Could you check a few things on this model? Use its own coordinates, in mm. Face numbers are marked on the shaded views. A direction names the side the tool comes from. Coordinates: 2 decimals unless noted, no trailing zeros. Loops run counter-clockwise (first coordinate to the right, second up) from the corner with the lowest first, then second, coordinate; pieces in that order, holes last. Notation, with made-up numbers: M -33.5,-40 L -12.5,-40 A11 ccw -12.5,-24 Z; hole C 53.5,-13.5 d11. An arc over 180 degrees is marked long. Write each question's results on one line, items separated by ' | '.
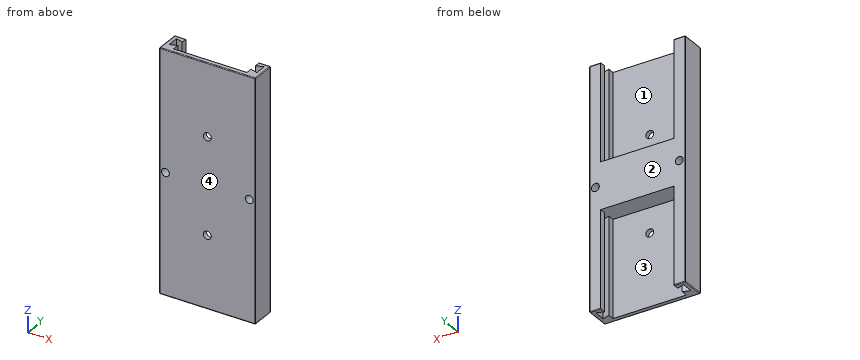
Autodesk Inventor part; units mm, degrees
ref_plane "YZ Plane" through (0, 0, 0) normal (1, 0, 0) x (0, 1, 0)
ref_plane "XZ Plane" through (0, 0, 0) normal (0, 1, 0) x (-1, 0, 0)
ref_plane "XY Plane" through (0, 0, 0) normal (0, 0, 1) x (1, 0, 0)
sketch "Sketch1" plane through (0, 0, 0) normal (0, 0, 1) x (1, 0, 0)
  line L0 (0, 0) -> (40, 0)
  line L1 (40, 0) -> (40, 10)
  line L2 (40, 10) -> (0, 10)
  line L3 (0, 10) -> (0, 0)
  dimension "d0" = 40
  dimension "d1" = 10
extrude "Extrusion1" add sketch "Sketch1" against normal blind 100
sketch "Sketch2" plane through (0, 0, 0) normal (0, 0, 1) x (1, 0, 0)
  line L0 (4.7, 1.898) -> (35.3, 1.898)
  line L1 (38.3, 8.5152) -> (38.3, 3.6828)
  line L2 (1.7, 8.5152) -> (1.7, 3.6828)
  line L3 (35.3, 7.5152) -> (38.3, 8.5152)
  line L4 (35.3, 7.5152) -> (35.3, 10)
  line L5 (35.3, 1.898) -> (35.3, 4.6828)
  line L6 (38.3, 3.6828) -> (35.3, 4.6828)
  line L7 (4.7, 7.5152) -> (1.7, 8.5152)
  line L8 (4.7, 10) -> (4.7, 7.5152)
  line L9 (4.7, 4.6828) -> (4.7, 1.898)
  line L10 (1.7, 3.6828) -> (4.7, 4.6828)
  line L11 (4.7, 10) -> (35.3, 10)
extrude "Extrusion2" cut sketch "Sketch2" against normal blind 40.3
sketch "Sketch3" plane through (0, 0, -100) normal (0, 0, -1) x (-1, 0, 0)
  line L0 (-35.3, 1.898) -> (-4.7, 1.898)
  line L1 (-1.7, 8.5152) -> (-1.7, 3.6828)
  line L2 (-38.3, 8.5152) -> (-38.3, 3.6828)
  line L3 (-4.7, 7.5152) -> (-1.7, 8.5152)
  line L4 (-4.7, 7.5152) -> (-4.7, 10)
  line L5 (-4.7, 1.898) -> (-4.7, 4.6828)
  line L6 (-1.7, 3.6828) -> (-4.7, 4.6828)
  line L7 (-35.3, 7.5152) -> (-38.3, 8.5152)
  line L8 (-35.3, 10) -> (-35.3, 7.5152)
  line L9 (-35.3, 4.6828) -> (-35.3, 1.898)
  line L10 (-38.3, 3.6828) -> (-35.3, 4.6828)
  line L11 (-35.3, 10) -> (-4.7, 10)
extrude "Extrusion3" cut sketch "Sketch3" against normal blind 40.3
sketch "Sketch5" plane through (4.7, 1.898, 0) normal (0, 1, 0) x (1, 0, 0)
  circle A0 centre (15.3, 30) radius 1.65
  line L0 (35.3, 0) -> (35.3, 100)
  circle A1 centre (15.3, 70) radius 1.65
  point P0 (-4.7, 0)
extrude "Extrusion5" cut sketch "Sketch5" against normal blind 5
fillet "Fillet1" radius 0.3 14 edges at (2.35, 10, -100) (37.65, 10, -100) (0, 5, -100) (0, 10, -50) (0, 0, -50) (20, 0, -100) (40, 5, -100) (0, 5, 0) (40, 10, -50) (40, 0, -50) (20, 0, 0) (40, 5, 0) (2.35, 10, 0) (37.65, 10, 0)
sketch "Sketch6" plane through (4.7, 10, -40.3) normal (0, 1, 0) x (1, 0, 0)
  line L0 (-4.4, -40) -> (-4.4, 59.4)
  line L1 (-4.7, 59.4) -> (-4.7, -40)
  line L2 (35.3, -40) -> (35.3, 59.4)
  circle A0 centre (32.8, 9.7) radius 1.65
  circle A1 centre (-2.2, 9.7) radius 1.65
  point P0 (-4.7, -40.3)
  dimension "d29" = 3.3
  dimension "d30" = 3.3
extrude "Extrusion6" cut sketch "Sketch6" against normal blind 10
properties part number "centralBody"
(1) Imagine slicing it at C-C, the plane z = -50. List the corners of the cut face in (x, y) for me.
Reported:
outline: M 0,0.3 A0.3 ccw 0.3,0 L 0.85,0 L 0.85,10 L 0.3,10 A0.3 ccw 0,9.7 Z; M 4.15,0 L 35.85,0 L 35.85,10 L 4.15,10 Z; M 39.15,0 L 39.7,0 A0.3 ccw 40,0.3 L 40,9.7 A0.3 ccw 39.7,10 L 39.15,10 Z
(2) Please list where these lines run through material, in increasing order: probe 1 along X at (y, z) = (8, -50); probe 2 along Z at (x, y) = (20, 1.45); probe 3 along X at (y, z) = (1.3, -70). Write a range as from..to.
Reported:
probe 1: x = 0..0.85, 4.15..35.85, 39.15..40 | probe 2: z = -100..-71.65, -68.35..-31.65, -28.35..0 | probe 3: x = 0..18.35, 21.65..40
(3) Which directions (+Z, -Z, +X, -X, +Y, -Y) give clear straight access to the entire face, cutting with the end or side of a thin tool? Please do the marked faces 3 and 4.
Reported:
face 3: -Z, +Y | face 4: +Z, -Z, +X, -X, -Y
(4) Will these pins go through, and if not, where does the flat tip stop? P1, Ø3, axis at x = 10.5, z = -28.5, coming from the +Y side; P2, Ø1.5, axis at x = 11, y = 4.5, coming from the -Z side; P3, Ø2.5, axis at y = 5.5, z = -17, coming from the -X side; P4, Ø2.5, axis at x = 26, y = 7, coming from the +Z side.
Reported:
P1: stops at y = 1.9 | P2: stops at z = -59.7 | P3: stops at x = 0 | P4: stops at z = -40.3
(5) Imagine slicing it at B-B, the plane x = 20. List the corners of the cut face in (y, z) for me, and give its area (3 significant figures).
Reported:
outline: M 0,-99.7 A0.3 ccw 0.3,-100 L 1.9,-100 L 1.9,-71.65 L 0,-71.65 Z; M 0,-68.35 L 1.9,-68.35 L 1.9,-59.7 L 10,-59.7 L 10,-40.3 L 1.9,-40.3 L 1.9,-31.65 L 0,-31.65 Z; M 0,-28.35 L 1.9,-28.35 L 1.9,0 L 0.3,0 A0.3 ccw 0,-0.3 Z | area: 334 mm2
(6) Imagine slicing it at A-A, the plane z = -70. List the corners of the cut face in (x, y) for me.
Reported:
outline: M 0,0.3 A0.3 ccw 0.3,0 L 18.35,0 L 18.35,1.9 L 4.7,1.9 L 4.7,4.68 L 1.7,3.68 L 1.7,8.52 L 4.7,7.52 L 4.7,10 L 0.3,10 A0.3 ccw 0,9.7 Z; M 21.65,0 L 39.7,0 A0.3 ccw 40,0.3 L 40,9.7 A0.3 ccw 39.7,10 L 35.3,10 L 35.3,7.52 L 38.3,8.52 L 38.3,3.68 L 35.3,4.68 L 35.3,1.9 L 21.65,1.9 Z
(7) If we mould it in two halves opening along X, with no side actions, what happens to the marked faces 1 and 2? For each: released by +X, released by -X, zero draft, split by the parting line, or undercut.
Reported:
face 1: undercut | face 2: zero draft
(8) Imagine slicing it at D-D, the plane y = 6. List the corners of the cut face in (x, z) for me, and give its area (3 significant figures).
Reported:
outline: M 0,-99.7 A0.3 ccw 0.3,-100 L 1.7,-100 L 1.7,-59.7 L 38.3,-59.7 L 38.3,-100 L 39.7,-100 A0.3 ccw 40,-99.7 L 40,-0.3 A0.3 ccw 39.7,0 L 38.3,0 L 38.3,-40.3 L 1.7,-40.3 L 1.7,0 L 0.3,0 A0.3 ccw 0,-0.3 Z; hole C 2.5,-50 d3.3; hole C 37.5,-50 d3.3 | area: 1,030 mm2
